from build123d import *

# Parameters (mm, degrees)
BOSS_EXTRUDE1_DEPTH = 4
SKETCH2_R           = 0.75
CUT_EXTRUDE1_DEPTH  = 4
SKETCH4_R           = 0.75
CUT_EXTRUDE2_DEPTH  = 2
CUT_EXTRUDE3_START  = -3
SKETCH4_3_R         = 0.75
CUT_EXTRUDE3_DEPTH  = 1


with BuildPart() as part:
    # Sketch1 → Boss-Extrude1 (new body)
    with BuildSketch(Plane.XY):
        with BuildLine():
            Line((-10.44, 2), (10.44, 2))
            ThreePointArc((10.44, 2), (12.44, 0), (10.44, -2))
            Line((10.44, -2), (-10.44, -2))
            ThreePointArc((-10.44, -2), (-12.44, 0), (-10.44, 2))
        make_face()
    extrude(amount=BOSS_EXTRUDE1_DEPTH)

    # Sketch2 → Cut-Extrude1 (cut)
    with BuildSketch(Plane.XY.offset(4)):
        with Locations((-10.44, 0)):
            Circle(SKETCH2_R)
        with Locations((10.44, 0)):
            Circle(SKETCH2_R)
    extrude(amount=-CUT_EXTRUDE1_DEPTH, mode=Mode.SUBTRACT)

    # Sketch4 → Cut-Extrude2 (cut)
    # profile 1 of 2: a face of its own
    with BuildSketch(Plane.XY.offset(4)):
        with BuildLine():
            ThreePointArc((-6.99, -2), (-8.99, 0), (-6.99, 2))
            Line((-6.99, 2), (-10.44, 2))
            ThreePointArc((-10.44, 2), (-12.44, 0), (-10.44, -2))
            Line((-10.44, -2), (-6.99, -2))
        make_face()
        with Locations((-10.44, 0)):
            Circle(SKETCH4_R, mode=Mode.SUBTRACT)
    # profile 2 of 2: a face of its own
    with BuildSketch(Plane.XY.offset(4)):
        with BuildLine():
            Line((10.44, 2), (6.99, 2))
            ThreePointArc((6.99, 2), (8.99, 0), (6.99, -2))
            Line((6.99, -2), (10.44, -2))
            ThreePointArc((10.44, -2), (12.44, 0), (10.44, 2))
        make_face()
        with Locations((10.44, 0)):
            Circle(SKETCH4_R, mode=Mode.SUBTRACT)
    extrude(amount=-CUT_EXTRUDE2_DEPTH, mode=Mode.SUBTRACT)

    # Sketch4<3> → Cut-Extrude3 (cut)
    # profile 1 of 2: a face of its own
    with BuildSketch(Plane.XY.offset(4).offset(CUT_EXTRUDE3_START)):
        with BuildLine():
            ThreePointArc((-6.99, -2), (-8.99, 0), (-6.99, 2))
            Line((-6.99, 2), (-10.44, 2))
            ThreePointArc((-10.44, 2), (-12.44, 0), (-10.44, -2))
            Line((-10.44, -2), (-6.99, -2))
        make_face()
        with Locations((-10.44, 0)):
            Circle(SKETCH4_3_R, mode=Mode.SUBTRACT)
    # profile 2 of 2: a face of its own
    with BuildSketch(Plane.XY.offset(4).offset(CUT_EXTRUDE3_START)):
        with BuildLine():
            Line((10.44, 2), (6.99, 2))
            ThreePointArc((6.99, 2), (8.99, 0), (6.99, -2))
            Line((6.99, -2), (10.44, -2))
            ThreePointArc((10.44, -2), (12.44, 0), (10.44, 2))
        make_face()
        with Locations((10.44, 0)):
            Circle(SKETCH4_3_R, mode=Mode.SUBTRACT)
    extrude(amount=-CUT_EXTRUDE3_DEPTH, mode=Mode.SUBTRACT)


solid = part.part
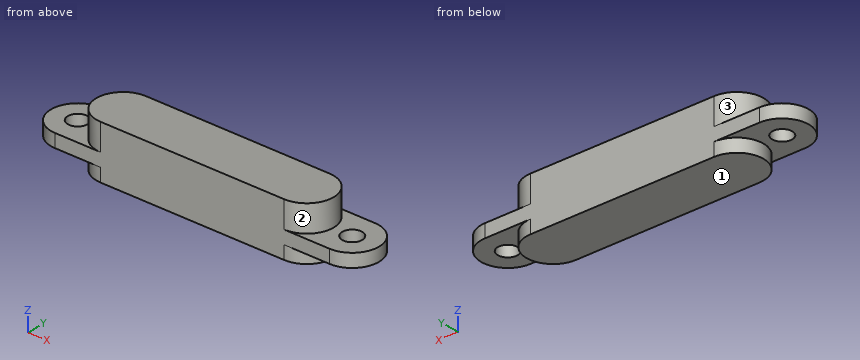
Could you check a few things on this model? Use its own coordinates, in mm. Face numbers are marked on the shaded views. A direction names the side the tool comes from. Give positions to 0.01 mm unless a question says otherwise; leave off trailing zeros. Order: outer loops, then holes, each group sorted by start corner. A loop starts at its lowest first (then second) coordinate and runs counter-clockwise, first axis right, second up.
1. For the marked faces 1, 2 and 3, which set-ups out of +Z, -Z, +X, -X, +Y, -Y let a thin tool reach every point of the face, with its end or its side?
2. Will these pins go through, and if not, where does the flat tip stop? P1, Ø1.2, axis at x = 11, y = 1, coming from the -Z side; P2, Ø1.5, axis at y = 1.5, z = 0.5, coming from the -X side.
3. Suppose I cut it at A-A (y = 0.4). List the corners of the cut face in (x, z) for me.
4. Suppose I cut it at B-B (x = -10). List the corners of the cut face in (y, z) for me.
5. Suppose I cut it at D-D (z = 0.7). List the corners of the cut face in (x, y) for me, plus the area to 3 significant figures.
6. Suppose I cut it at C-C (y = -1.3). List the corners of the cut face in (x, z) for me.
7. I need wall thicknesses on L1, parallel to Y at x = -10.44, z = 1.4; L2, parallel to Z at x = -9.25, y = -1.75; L3, parallel to X at y = 0.15, z = 1.2. Which ranges of each line are inside material? Lowest first, please.
Solved:
1. face 1: -Z, +X, -X, +Y, -Y
1. face 2: +Z, +X
1. face 3: +Z, -X
2. P1: stops at z = 1
2. P2: stops at x = -12.2
3. outline: (-12.4, 1) - (-11.07, 1) - (-11.07, 2) - (-12.4, 2) - close; (-9.81, 1) - (-8.95, 1) - (-8.95, 0) - (8.95, 0) - (8.95, 1) - (9.81, 1) - (9.81, 2) - (8.95, 2) - (8.95, 4) - (-8.95, 4) - (-8.95, 2) - (-9.81, 2) - close; (11.07, 1) - (12.4, 1) - (12.4, 2) - (11.07, 2) - close
4. outline: (-2, 1) - (-0.61, 1) - (-0.61, 2) - (-2, 2) - close; (0.61, 1) - (2, 1) - (2, 2) - (0.61, 2) - close
5. outline: (-6.99, -2) - (6.99, -2) arc R2 ccw to (6.99, 2) - (-6.99, 2) arc R2 ccw to start
5. area: 68.5 mm2
6. outline: (-11.96, 1) - (-8.51, 1) - (-8.51, 0) - (8.51, 0) - (8.51, 1) - (11.96, 1) - (11.96, 2) - (8.51, 2) - (8.51, 4) - (-8.51, 4) - (-8.51, 2) - (-11.96, 2) - close
7. L1: y = -2 to -0.75, 0.75 to 2
7. L2: z = 1 to 2
7. L3: x = -12.43 to -11.17, -9.71 to 9.71, 11.17 to 12.43
